Geometry: final body of the model. Coordinates: model frame, mm. Round coordinates to 2 decimals unless told otherwise and drop trailing zeros. Write each loop counter-clockwise with the first axis right and the second up, starting at its lowest first coordinate (ties: lowest second). Pieces come first, ordered by that corner, then holes. Notation, with made-up numbers: M -27.5,-4.75 L -20.5,-4.75 A18 cw -20.5,11.25 Z; hole C 5,24 d2. An arc over 180 degrees is marked long. Answer as CSV lines item,"result". Start each with the question number.
Q1. Ray query, probe 1 along X at (y, z) = (-87.5, 1.5); probe 2 along X at (y, z) = (-65.5, 1.9); probe 3 along Y at (x, z) = (-18, 0.75). Return the intervals inside material, ascending.
Q2. Section query C-C on z = 1.65. Give the number of separate pieces and of enclosed holes in the cut face, and give its area (3 significant figures).
Q3. Section query A-A on y = -88. Output: boundary loops of the cut face in (x, z) (3 decimals).
Q4. Section query B-B on x = 58. Output: boundary loops of the cut face in (y, z) (3 decimals).
Q5. First-contact query: pin 1 (1 mm diameter, centred on x = 58, z = 2, fed in from +Y); pin 2 (1.6 mm diameter, centred on x = -21.5, z = 2, fed in from -Y); pin 3 (2.5 mm diameter, centred on x = 112.5, y = -92.1, fed in from -Z); pin 4 (1 mm diameter, centred on y = -93, z = 1.5, fed in from -X). Flat tips, straight axial feed; report the tip coordinate or a pass-through.
```python
from build123d import *

# Parameters (mm, degrees)
SKETCH1_W               = 200
SKETCH1_H               = 127
BOSS_EXTRUDE1_DEPTH     = 3.175
SKETCH4_W               = 11.35
SKETCH4_H               = 13.0800094
SKETCH4_W_2             = 86.049970282
SKETCH4_W_3             = 11.50001
SKETCH4_W_4             = 86.500000282
CUT_EXTRUDE1_DEPTH      = 4.175
SKETCH5_R               = 6
CUT_EXTRUDE2_DEPTH      = 1
CUT_EXTRUDE2_DEPTH_BACK = 4.175
SKETCH6_R               = 1.7145
CUT_EXTRUDE3_DEPTH      = 4.175


with BuildPart() as part:
    # Sketch1 → Boss-Extrude1 (new body)
    with BuildSketch(Plane.XY):
        with Locations((52.222222222, -34.055555556)):
            Rectangle(SKETCH1_W, SKETCH1_H)
    extrude(amount=BOSS_EXTRUDE1_DEPTH)

    # Sketch4 → Cut-Extrude1 (cut, through all)
    with BuildSketch(Plane(origin=(0, 0, 0), x_dir=(-1, 0, 0), z_dir=(0, 0, -1))):
        with Locations((-146.547222222, 22.904439744)):
            Rectangle(SKETCH4_W, SKETCH4_H)
        with Locations((-123.847222222, 22.904439744)):
            Rectangle(SKETCH4_W, SKETCH4_H)
        with Locations((-63.797237175, 22.904439744)):
            Rectangle(SKETCH4_W_2, SKETCH4_H)
        with Locations((-3.672247128, 22.904439744)):
            Rectangle(SKETCH4_W_3, SKETCH4_H)
        with Locations((19.177762872, 22.904439744)):
            Rectangle(SKETCH4_W_3, SKETCH4_H)
        with Locations((42.027772778, 22.904439744)):
            Rectangle(SKETCH4_W_3, SKETCH4_H)
        with Locations((-146.547222222, -91.015550856)):
            Rectangle(SKETCH4_W, SKETCH4_H)
        with Locations((-123.847222222, -91.015550856)):
            Rectangle(SKETCH4_W, SKETCH4_H)
        with Locations((-63.572222175, -91.015550856)):
            Rectangle(SKETCH4_W_4, SKETCH4_H)
        with Locations((-3.297222034, -91.015550856)):
            Rectangle(SKETCH4_W, SKETCH4_H)
        with Locations((19.402777872, -91.015550856)):
            Rectangle(SKETCH4_W, SKETCH4_H)
        with Locations((42.102777778, -91.015550856)):
            Rectangle(SKETCH4_W, SKETCH4_H)
    extrude(amount=-CUT_EXTRUDE1_DEPTH, mode=Mode.SUBTRACT)

    # Sketch5 → Cut-Extrude2 (cut, two sides)
    with BuildSketch(Plane(origin=(0, 0, 0), x_dir=(-1, 0, 0), z_dir=(0, 0, -1))) as cut_extrude2_sk:
        with Locations((-128.747542222, -65.425546156)):
            Circle(SKETCH5_R)
        with Locations((24.303097778, -65.425546156)):
            Circle(SKETCH5_R)
    extrude(amount=CUT_EXTRUDE2_DEPTH, mode=Mode.SUBTRACT)
    extrude(cut_extrude2_sk.sketch, amount=-CUT_EXTRUDE2_DEPTH_BACK, mode=Mode.SUBTRACT)

    # Sketch6 → Cut-Extrude3 (cut, through all)
    with BuildSketch(Plane(origin=(0, 0, 0), x_dir=(-1, 0, 0), z_dir=(0, 0, -1))):
        with Locations((-135.197222222, 23.984435044)):
            Circle(SKETCH6_R)
        with Locations((-112.497222269, 23.984435044)):
            Circle(SKETCH6_R)
        with Locations((-15.097252081, 23.984435044)):
            Circle(SKETCH6_R)
        with Locations((7.752757872, 23.984435044)):
            Circle(SKETCH6_R)
        with Locations((30.602767825, 23.984435044)):
            Circle(SKETCH6_R)
        with Locations((-112.497222269, -92.095546156)):
            Circle(SKETCH6_R)
        with Locations((-135.197222222, -92.095546156)):
            Circle(SKETCH6_R)
        with Locations((-14.647222034, -92.095546156)):
            Circle(SKETCH6_R)
        with Locations((8.052777919, -92.095546156)):
            Circle(SKETCH6_R)
        with Locations((30.752777825, -92.095546156)):
            Circle(SKETCH6_R)
    extrude(amount=-CUT_EXTRUDE3_DEPTH, mode=Mode.SUBTRACT)


solid = part.part
```
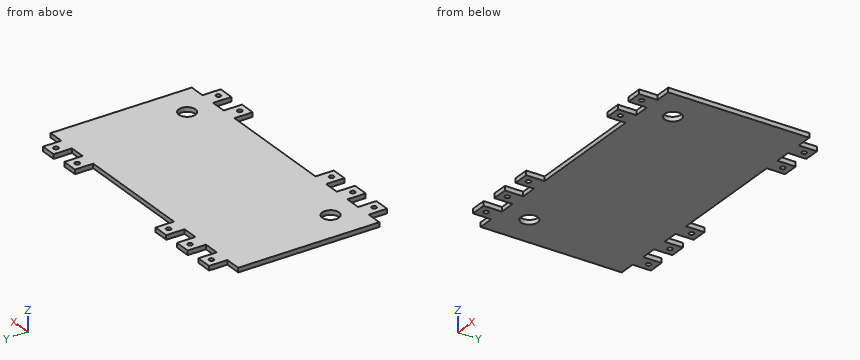
Entries:
1,probe 1,"x = -36.43 to -25.08, -13.73 to -2.38, 8.97 to 20.32, 106.82 to 118.17, 129.52 to 140.87"
1,probe 2,"x = -47.78 to -30.3, -18.3 to 122.75, 134.75 to 152.22"
1,probe 3,"y = -84.48 to 16.36"
2,separate pieces,"1"
2,enclosed holes,"12"
2,area,"21,300 mm^2"
3,outline,"M -36.428,0 L -25.078,0 L -25.078,3.175 L -36.428,3.175 Z; M -13.728,0 L -2.378,0 L -2.378,3.175 L -13.728,3.175 Z; M 8.972,0 L 20.322,0 L 20.322,3.175 L 8.972,3.175 Z; M 106.822,0 L 118.172,0 L 118.172,3.175 L 106.822,3.175 Z; M 129.522,0 L 140.872,0 L 140.872,3.175 L 129.522,3.175 Z"
4,outline,"M -84.476,0 L 16.364,0 L 16.364,3.175 L -84.476,3.175 Z"
5,pin 1,"stops at y = 16.36"
5,pin 2,"stops at y = -84.48"
5,pin 3,"passes through"
5,pin 4,"stops at x = -36.43"
